Read the model definition and answer for the solid it produces. Units are mm, in the model's axes. Coordinates: 2 decimals unless noted, no trailing zeros. Write each loop counter-clockwise with the first axis right and the second up, starting at its lowest first coordinate (ties: lowest second). Pieces come first, ordered by that corner, then holes. Notation, with made-up numbers: (-9, 48.5) -> (16, 48.5) arc R20 cw to (16, 66.5) -> close; hole circle Ø2 at (-19, 53). An arc over 180 degrees is marked (long way). Return JSON: item names as keys, results as strings.
from build123d import *

# Parameters (mm, degrees)
SCHIZZO1_W                   = 5
SCHIZZO1_H                   = 70
ESTRUSIONE_ESTRUSIONE1_DEPTH = 70
ESTRUSIONE_ESTRUSIONE2_START = -35
ESTRUSIONE_ESTRUSIONE2_DEPTH = 5
SCHIZZO3_R                   = 2.5
ESTRUSIONE_ESTRUSIONE3_DEPTH = 5
SCHIZZO4_W                   = 130
SCHIZZO4_H                   = 70
ESTRUSIONE_ESTRUSIONE4_DEPTH = 5
SCHIZZO5_R                   = 1.25
TAGLIO_ESTRUSIONE1_DEPTH     = 46
ESTRUSIONE_ESTRUSIONE5_DEPTH = 3
RACCORDO1_R                  = 5
RACCORDO2_R                  = 5
RACCORDO3_R                  = 2
RACCORDO4_R                  = 2
TAGLIO_ESTRUSIONE2_REACH     = 75


with BuildPart() as part:
    # Schizzo1 → Estrusione-Estrusione1 (new body)
    with BuildSketch(Plane.XY):
        with Locations((-2.5, 35)):
            Rectangle(SCHIZZO1_W, SCHIZZO1_H)
    extrude(amount=ESTRUSIONE_ESTRUSIONE1_DEPTH)

    # Schizzo2 → Estrusione-Estrusione2 (add)
    with BuildSketch(Plane.XY.offset(70).offset(ESTRUSIONE_ESTRUSIONE2_START)):
        with BuildLine():
            Line((0, 50), (0, 45))
            Line((0, 45), (7.531619243, 45))
            ThreePointArc((7.531619243, 45), (12.531619243, 50), (7.531619243, 55))
            Line((7.531619243, 55), (0, 55))
            Line((0, 55), (0, 50))
        make_face()
        with BuildLine():
            Line((0, 20), (0, 15))
            Line((0, 15), (7.531619243, 15))
            ThreePointArc((7.531619243, 15), (12.531619243, 20), (7.531619243, 25))
            Line((7.531619243, 25), (0, 25))
            Line((0, 25), (0, 20))
        make_face()
    extrude(amount=-ESTRUSIONE_ESTRUSIONE2_DEPTH)

    # Schizzo3 → Estrusione-Estrusione3 (add)
    with BuildSketch(Plane(origin=(0, 0, 30), x_dir=(-1, 0, 0), z_dir=(0, 0, -1))):
        with Locations((-7.547600082, 50.061310314)):
            Circle(SCHIZZO3_R)
        with Locations((-7.547600082, 19.939772921)):
            Circle(SCHIZZO3_R)
    extrude(amount=ESTRUSIONE_ESTRUSIONE3_DEPTH)

    # Schizzo4 → Estrusione-Estrusione4 (add)
    with BuildSketch(Plane.XZ):
        with Locations((60, 35)):
            Rectangle(SCHIZZO4_W, SCHIZZO4_H)
    extrude(amount=ESTRUSIONE_ESTRUSIONE4_DEPTH)

    # Schizzo5 → Taglio-Estrusione1 (cut, through all)
    with BuildSketch(Plane(origin=(0, 0, 25), x_dir=(-1, 0, 0), z_dir=(0, 0, -1))):
        with Locations((-7.547600082, 50.061310314)):
            Circle(SCHIZZO5_R)
        with Locations((-7.547600082, 19.939772921)):
            Circle(SCHIZZO5_R)
    extrude(amount=-TAGLIO_ESTRUSIONE1_DEPTH, mode=Mode.SUBTRACT)

    # Schizzo6 → Estrusione-Estrusione5 (add)
    with BuildSketch(Plane.XY.offset(70)):
        Polygon((125, 0), (0, 0), (0, 70), (-5, 70), (-5, -5), (125, -5), align=None)
        Polygon((0, 70), (125, 0), (0, 0), align=None)
    extrude(amount=ESTRUSIONE_ESTRUSIONE5_DEPTH)

    # Raccordo1
    raccordo1_edges = [part.edges().sort_by_distance(p)[0] for p in [
        (0, 35, 70),
        (62.5, 0, 70),
        (0, 0, 35),
    ]]
    fillet(raccordo1_edges, radius=RACCORDO1_R)

    # Raccordo2
    raccordo2_edges = [part.edges().sort_by_distance(p)[0] for p in [
        (0, 50, 35),
        (0, 20, 35),
    ]]
    fillet(raccordo2_edges, radius=RACCORDO2_R)

    # Raccordo3
    raccordo3_edges = [part.edges().sort_by_distance(p)[0] for p in [
        (0, 50, 30),
        (0, 20, 30),
    ]]
    fillet(raccordo3_edges, radius=RACCORDO3_R)

    # Raccordo4
    raccordo4_edges = [part.edges().sort_by_distance(p)[0] for p in [
        (0, 25, 32.5),
        (0, 15, 32.5),
        (0, 45, 32.5),
        (0, 55, 32.5),
    ]]
    fillet(raccordo4_edges, radius=RACCORDO4_R)

    # Schizzo7 → Taglio-Estrusione2 (cut, up to next)
    with BuildSketch(Plane(origin=(0, 0, 73), x_dir=(-1, 0, 0), z_dir=(0, 0, -1)), mode=Mode.PRIVATE) as taglio_estrusione2_sk1:
        with BuildLine():
            ThreePointArc((-5, 0), (-1.464466094, 1.464466094), (0, 5))
            Line((0, 5), (0, 70))
            Line((0, 70), (-125, 0))
            Line((-125, 0), (-5, 0))
        make_face()
    taglio_estrusione2_tool1 = extrude(taglio_estrusione2_sk1.sketch, amount=TAGLIO_ESTRUSIONE2_REACH, mode=Mode.PRIVATE) & part.part
    add(taglio_estrusione2_tool1.solids().sort_by_distance((41.716454, 23.360611, 73))[0], mode=Mode.SUBTRACT)


solid = part.part
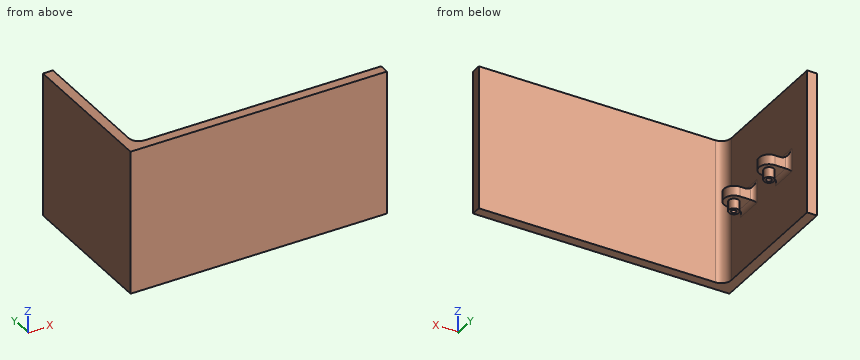
1. Consider L1, parallel to X at y = 23, z = 49.5; L2, parallel to X at y = 46, z = 36.5. Determine where each line is inside the solid, lowest interval first.
Taken from the geometry:
{"L1": "x = -5 to 0", "L2": "x = -5 to 1.43"}
2. The part is cut by section B-B (x = 43). Determine the outline of the cut face in (y, z).
Taken from the geometry:
{"outline": "(-5, 0) -> (0, 0) -> (0, 73) -> (-5, 73) -> close"}
3. The part is cut by section A-A (z = 47.5). Determine the outline of the cut face in (x, y).
Taken from the geometry:
{"outline": "(-5, -5) -> (125, -5) -> (125, 0) -> (5, 0) arc R5 cw to (0, 5) -> (0, 70) -> (-5, 70) -> close"}
4. Flat-ended cylindrical pins translate along their axes: pin 1 Ø8 at (x, z) = (66, 17) entering from +Y; pin 2 Ø8.5 at (x, y) = (8.5, 50.5) entering from +Z; pin 3 Ø2 at (x, y) = (7.55, 19.94) entering from -Z; pin 4 Ø4 at (x, y) = (7, 19) entering from -Z. Find the tip coordinate at first contact, or state that the pin passes through.
Taken from the geometry:
{"pin 1": "stops at y = 0", "pin 2": "stops at z = 35.06", "pin 3": "passes through", "pin 4": "stops at z = 25"}
